Check sheet for the modelled part. Datum: model origin and axes. Units: mm. Face numbers are marked on the shaded views. A direction names the side the tool comes from. Round coordinates to 2 decimals unless told otherwise and drop trailing zeros. Write each loop counter-clockwise with the first axis right and the second up, starting at its lowest first coordinate (ties: lowest second). Pieces come first, ordered by that corner, then holes.
Item 1: Go/stop test with flat-tipped pins: pin 1 Ø6 at (x, z) = (-8, -12.5) entering from +Y; pin 2 Ø8 at (x, z) = (-8, -23.5) entering from -Y; pin 3 Ø4 at (x, y) = (-2.5, 11.5) entering from -Z. Record where each tip stops, or that it passes through.
Item 2: Cross-section at C-C on z = -11.5. Enter the section's corners in (x, y), plus the area to 3 significant figures.
Item 3: Material ranges on line 1 (Y direction, x = -20.25, z = -22); line 2 (Z direction, x = -8.75, y = 18), recorded low to high.
Item 4: Tool access check on the marked faces 1 and 2. Record the directions out of +Z, -Z, +X, -X, +Y, -Y that give a thin tool (end or side, any length) a straight path to the whole face; none if there is none.
Item 5: Cross-section at A-A on x = -19. Enter the section's corners in (y, z), plus the area to 3 significant figures.
Item 6: Cross-section at B-B on y = 6. Enter the section's corners in (x, z).
Item 7: Cross-section at D-D on x = -9.25. Enter the section's corners in (y, z).
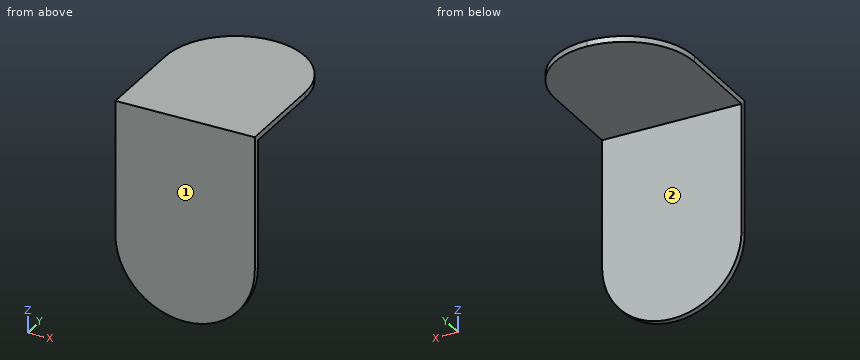
Autodesk Inventor part; units mm, degrees
ref_plane "YZ Plane" through (0, 0, 0) normal (1, 0, 0) x (0, 1, 0)
ref_plane "XZ Plane" through (0, 0, 0) normal (0, 1, 0) x (-1, 0, 0)
ref_plane "XY Plane" through (0, 0, 0) normal (0, 0, 1) x (1, 0, 0)
sketch "Sketch1" plane through (0, 0, 0) normal (0, 1, 0) x (-1, 0, 0)
  line L0 (0, 0) -> (24, 0)
  line L1 (24, 0) -> (24, -35)
  line L2 (0, -35) -> (0, 0)
  arc A0 (0, -23) -> (24, -23) centre (12, -23) ccw
  dimension "d0" = 24
  dimension "d1" = 35
extrude "Extrusion1" add sketch "Sketch1" along normal blind 1
sketch "Sketch2" plane through (0, 1, 0) normal (0, 1, 0) x (1, 0, 0)
  line L0 (-24, 0) -> (0, 0)
  line L1 (0, 0) -> (0, 23)
  line L2 (-24, 0) -> (0, 0)
  line L3 (0, 0) -> (0, 1)
  line L4 (0, 1) -> (-24, 1)
  line L5 (-24, 1) -> (-24, 0)
  dimension "d4" = 1
extrude "Extrusion2" add sketch "Sketch2" along normal blind 27
fillet "Fillet1" radius 12 2 edges at (0, 28, -0.5) (-24, 28, -0.5)
properties part number "linkage connector"
Response values:
1. pin 1: stops at y = 1
1. pin 2: stops at y = 0
1. pin 3: stops at z = -1
2. outline: (-24, 0) - (0, 0) - (0, 1) - (-24, 1) - close
2. area: 24.0 mm2
3. line 1: y = 0 to 1
3. line 2: z = -1 to 0
4. face 1: +Z, -Z, +X, -X, -Y
4. face 2: -Z, +X, -X, +Y
5. outline: (0, -32.75) - (1, -32.75) - (1, -1) - (25.75, -1) - (25.75, 0) - (0, 0) - close
5. area: 57.5 mm2
6. outline: (-24, -1) - (0, -1) - (0, 0) - (-24, 0) - close
7. outline: (0, -34.68) - (1, -34.68) - (1, -1) - (27.68, -1) - (27.68, 0) - (0, 0) - close
